```python
from build123d import *

# Parameters (mm, degrees)
F1_DEPTH = 5


with BuildPart() as f1:
    # F0 (on Front) → F1 (new body)
    with BuildSketch(Plane.XZ):
        with BuildLine():
            ThreePointArc((-75, -29.5), (-72.656854, -35.156854), (-67, -37.5))
            Line((-67, -37.5), (-60.549265, -37.5))
            Line((-60.549265, -37.5), (-60.549265, 2.5))
            ThreePointArc((-60.549265, 2.5), (-58.499013, 7.449747), (-53.549265, 9.5))
            ThreePointArc((-53.549265, 9.5), (-48.599518, 7.449747), (-46.549265, 2.5))
            Line((-46.549265, 2.5), (-46.549265, -37.5))
            Line((-46.549265, -37.5), (67, -37.5))
            ThreePointArc((67, -37.5), (72.656854, -35.156854), (75, -29.5))
            Line((75, -29.5), (75, 29.5))
            ThreePointArc((75, 29.5), (72.656854, 35.156854), (67, 37.5))
            Line((67, 37.5), (60.549265, 37.5))
            Line((60.549265, 37.5), (60.549265, -2.5))
            ThreePointArc((60.549265, -2.5), (58.499013, -7.449747), (53.549265, -9.5))
            ThreePointArc((53.549265, -9.5), (48.599518, -7.449747), (46.549265, -2.5))
            Line((46.549265, -2.5), (46.549265, 37.5))
            Line((46.549265, 37.5), (-67, 37.5))
            ThreePointArc((-67, 37.5), (-72.656854, 35.156854), (-75, 29.5))
            Line((-75, 29.5), (-75, -29.5))
        make_face()
        with BuildLine():
            ThreePointArc((-21.549265, 12.5), (-18.620333, 19.571068), (-11.549265, 22.5))
            Line((-11.549265, 22.5), (11.549265, 22.5))
            ThreePointArc((11.549265, 22.5), (18.620333, 19.571068), (21.549265, 12.5))
            Line((21.549265, 12.5), (21.549265, -12.5))
            ThreePointArc((21.549265, -12.5), (18.620333, -19.571068), (11.549265, -22.5))
            Line((11.549265, -22.5), (-11.549265, -22.5))
            ThreePointArc((-11.549265, -22.5), (-18.620333, -19.571068), (-21.549265, -12.5))
            Line((-21.549265, -12.5), (-21.549265, 12.5))
        make_face(mode=Mode.SUBTRACT)
    extrude(amount=F1_DEPTH)


solid = f1.part
```
The listing builds one solid part. Answer for the finished solid, in the listing's coordinates (mm). A direction names the side the tool comes from. Round coordinates to 2 decimals unless told otherwise and drop trailing zeros. Loops run counter-clockwise (first coordinate to the right, second up) from the corner with the lowest first, then second, coordinate; pieces in that order, holes last. Notation, with made-up numbers: (45.5, -18.5) - (87.5, -18.5) arc R20 cw to (87.5, 18.5) - close; hole circle Ø11 at (51.5, -7). An arc over 180 degrees is marked (long way). Return JSON: item names as keys, results as strings. Group by question number.
1. The part is cut by section B-B on y = -3.7. Determine the outline of the cut face in (x, z), then the cut area to 3 significant figures.
2. Which of the six approach directions +Z, -Z, +X, -X, +Y, -Y give full straight-line access (tool end or side, diameter ignored) to faces 4 (the cylindrical face through (18.54, -2.46, 19.65)), 5 (the flat face through (-1, -5, -24)), 6 (the flat face through (46.549, -2, 17))?
3. The part is cut by section C-C on x = 10. Determine the outline of the cut face in (y, z), then the cut area to 3 significant figures.
4. The part is cut by section D-D on z = 19. Determine the outline of the cut face in (x, y).
5. The mould has two halves that part along X. Classify faces 1 (the flat face through (-75, -2, 0)), 2 (the flat face through (64, -2, 37.5)), 3 (the flat face through (-46.549, -2, -17)): pulls with the +X half, pulls with the -X half, needs draft (parallel to the pull), parting line crosses it, or undercut.
6. The part is cut by section A-A on z = -24. Determine the outline of the cut face in (x, y), then the cut area to 3 significant figures.
7. Consider probe 1 along Z at (x, y) = (-7.5, -3.7); probe 2 along X at (y, z) = (-0.55, 27.5); probe 3 along X at (y, z) = (-1.35, -11). Determine where each line is inside the solid, lowest interval first.
Resolved:
{
 "1": {"outline": "(-75, -29.5) arc R8 ccw to (-67, -37.5) - (-60.55, -37.5) - (-60.55, 2.5) arc R7 cw to (-53.55, 9.5) arc R7 cw to (-46.55, 2.5) - (-46.55, -37.5) - (67, -37.5) arc R8 ccw to (75, -29.5) - (75, 29.5) arc R8 ccw to (67, 37.5) - (60.55, 37.5) - (60.55, -2.5) arc R7 cw to (53.55, -9.5) arc R7 cw to (46.55, -2.5) - (46.55, 37.5) - (-67, 37.5) arc R8 ccw to (-75, 29.5) - close; hole (-21.55, -12.5) arc R10 ccw to (-11.55, -22.5) - (11.55, -22.5) arc R10 ccw to (21.55, -12.5) - (21.55, 12.5) arc R10 ccw to (11.55, 22.5) - (-11.55, 22.5) arc R10 ccw to (-21.55, 12.5) - close", "area": "8,070 mm²"},
 "2": {"face 4": "+Y, -Y", "face 5": "+Z, -Z, +X, -X, -Y", "face 6": "+Z, +Y, -Y"},
 "3": {"outline": "(-5, -37.5) - (0, -37.5) - (0, -22.5) - (-5, -22.5) - close; (-5, 22.5) - (0, 22.5) - (0, 37.5) - (-5, 37.5) - close", "area": "150 mm²"},
 "4": {"outline": "(-75, -5) - (-19.15, -5) - (-19.15, 0) - (-75, 0) - close; (19.15, -5) - (46.55, -5) - (46.55, 0) - (19.15, 0) - close; (60.55, -5) - (75, -5) - (75, 0) - (60.55, 0) - close"},
 "5": {"face 1": "pulls with the -X half", "face 2": "needs draft", "face 3": "undercut"},
 "6": {"outline": "(-75, -5) - (-60.55, -5) - (-60.55, 0) - (-75, 0) - close; (-46.55, -5) - (75, -5) - (75, 0) - (-46.55, 0) - close", "area": "680 mm²"},
 "7": {"probe 1": "z = -37.5 to -22.5, 22.5 to 37.5", "probe 2": "x = -75 to 46.55, 60.55 to 75", "probe 3": "x = -75 to -60.55, -46.55 to -21.55, 21.55 to 75"}
}
